```python
from build123d import *

# Parameters (mm, degrees)
SKETCH1_W           = 50
SKETCH1_H           = 40
SKETCH1_R           = 12.5
SKETCH1_R_2         = 2.75
SKETCH1_R_3         = 6
BOSS_EXTRUDE1_DEPTH = 2
SKETCH1_3_R         = 12.5
SKETCH1_3_R_2       = 6
BOSS_EXTRUDE2_DEPTH = 8
HOLE1_D             = 3
HOLE1_DEPTH         = 8
CIRPATTERN1_COUNT   = 4
FILLET1_R           = 10


with BuildPart() as part:
    # Sketch1 → Boss-Extrude1 (new body)
    with BuildSketch(Plane(origin=(0, 0, 0), x_dir=(1, 0, 0), z_dir=(0, 1, 0))):
        Rectangle(SKETCH1_W, SKETCH1_H)
        Circle(SKETCH1_R, mode=Mode.SUBTRACT)
        with Locations((-13.435028843, -13.435028843)):
            Circle(SKETCH1_R_2, mode=Mode.SUBTRACT)
        with Locations((-19, 0)):
            Circle(SKETCH1_R_2, mode=Mode.SUBTRACT)
        with Locations((-13.435028843, 13.435028843)):
            Circle(SKETCH1_R_2, mode=Mode.SUBTRACT)
        with Locations((13.435028843, 13.435028843)):
            Circle(SKETCH1_R_2, mode=Mode.SUBTRACT)
        with Locations((19, 0)):
            Circle(SKETCH1_R_2, mode=Mode.SUBTRACT)
        with Locations((13.435028843, -13.435028843)):
            Circle(SKETCH1_R_2, mode=Mode.SUBTRACT)
        Circle(SKETCH1_R)
        Circle(SKETCH1_R_3, mode=Mode.SUBTRACT)
    extrude(amount=BOSS_EXTRUDE1_DEPTH)

    # Sketch1<3> → Boss-Extrude2 (add)
    with BuildSketch(Plane(origin=(0, 0, 0), x_dir=(1, 0, 0), z_dir=(0, 1, 0))):
        Circle(SKETCH1_3_R)
        Circle(SKETCH1_3_R_2, mode=Mode.SUBTRACT)
    extrude(amount=BOSS_EXTRUDE2_DEPTH)

    # Hole1
    with Locations(Plane(origin=(0, 8, 0), x_dir=(1, 0, 0), z_dir=(0, 1, 0))):
        with Locations((0, -9.5)):
            hole1 = Hole(HOLE1_D / 2, depth=HOLE1_DEPTH)

    # CirPattern1: Hole1 ×4 about axis
    cirpattern1_axis = Axis((0, 0, 0), (0, 1, 0))
    for i in range(1, CIRPATTERN1_COUNT):
        add(hole1.rotate(cirpattern1_axis, i * 360 / CIRPATTERN1_COUNT), mode=Mode.SUBTRACT)

    # Fillet1
    fillet1_edges = [part.edges().sort_by_distance(p)[0] for p in [
        (25, 1, 20),
        (-25, 1, 20),
        (-25, 1, -20),
        (25, 1, -20),
    ]]
    fillet(fillet1_edges, radius=FILLET1_R)


solid = part.part
```
CAD build for the part. Positions are in the model's coordinates, mm. A direction names the side the tool comes from. Coordinates: 2 decimals unless noted, no trailing zeros. Loops run counter-clockwise (first coordinate to the right, second up) from the corner with the lowest first, then second, coordinate; pieces in that order, holes last. Notation, with made-up numbers: (21, 61) - (30, 61) arc R27 ccw to (30, 90) - close; hole circle Ø9 at (-11, 35.5). An arc over 180 degrees is marked (long way). Use CSV: the item, a comma, the result in double quotes. Start each with the question number.
Q1. Cut at B-B, the plane y = 5.25. List the corners of the cut face in (x, z), then the cut area to 3 significant figures.
Q2. Cut at D-D, the plane x = 4. List the corners of the cut face in (y, z).
Q3. Cut at A-A, the plane z = 0. List the corners of the cut face in (x, y).
Q4. Probe probe 1 along X at (y, z) = (4.75, 0); probe 2 along X at (y, z) = (5, 1). List the from-to ranges inside material, lowest first. Write a range as from..to.
Q5. Cut at C-C, the plane z = -14.5. List the corners of the cut face in (x, y), then the cut area to 3 significant figures.
Q6. Two-plate mould, pull along Z, no slides. Class faces 1 (the cylindrical face through (0, 4, -11)), 2 (the flat face through (25, 1, 0)), 3 (the flat face through (0, 1, -20)), 4 (the cylindrical face through (-22.15, 1.01, 16.99)): +Z half, -Z half, draft (parallel to the pull), parting line (faces both ways), or undercut.
Q7. 3-axis set-ups, long thin cutter, end or side, ignore diameter. For faces 5 (the cylindrical face through (21.99, 1.01, 17.15)), 6 (the flat face through (0, 2, -14)): which of +Z, -Z, +X, -X, +Y, -Y reach the whole face in a straight line?
Q8. Drop a flat-ended pin along its axis: P1, Ø6.5, axis at x = -19, z = 0, coming from the +Y side. Give the stop position or say it passes through.
Here are the results:
1,outline,"circle Ø25 at (0, 0); hole circle Ø3 at (-9.5, 0); hole circle Ø12 at (0, 0); hole circle Ø3 at (0, -9.5); hole circle Ø3 at (0, 9.5); hole circle Ø3 at (9.5, 0)"
1,area,"350 mm2"
2,outline,"(0, -20) - (2, -20) - (2, -11.84) - (8, -11.84) - (8, -4.47) - (0, -4.47) - close; (0, 4.47) - (8, 4.47) - (8, 11.84) - (2, 11.84) - (2, 20) - (0, 20) - close"
3,outline,"(-25, 0) - (-21.75, 0) - (-21.75, 2) - (-25, 2) - close; (-16.25, 0) - (-11, 0) - (-11, 8) - (-12.5, 8) - (-12.5, 2) - (-16.25, 2) - close; (-8, 0) - (-6, 0) - (-6, 8) - (-8, 8) - close; (6, 0) - (8, 0) - (8, 8) - (6, 8) - close; (11, 0) - (16.25, 0) - (16.25, 2) - (12.5, 2) - (12.5, 8) - (11, 8) - close; (21.75, 0) - (25, 0) - (25, 2) - (21.75, 2) - close"
4,probe 1,"-12.5..-11, -8..-6, 6..8, 11..12.5"
4,probe 2,"-12.46..-10.62, -8.38..-5.92, 5.92..8.38, 10.62..12.46"
5,outline,"(-23.93, 0) - (-15.97, 0) - (-15.97, 2) - (-23.93, 2) - close; (-10.9, 0) - (10.9, 0) - (10.9, 2) - (-10.9, 2) - close; (15.97, 0) - (23.93, 0) - (23.93, 2) - (15.97, 2) - close"
5,area,"75.4 mm2"
6,face 1,"undercut"
6,face 2,"draft"
6,face 3,"-Z half"
6,face 4,"+Z half"
7,face 5,"+Z, +X, +Y, -Y"
7,face 6,"+Y"
8,P1,"y = 2"
